Design review of the part built by this model. Coordinates are the model's own, in mm. Round coordinates to 2 decimals unless told otherwise and drop trailing zeros. Loops run counter-clockwise (first coordinate to the right, second up) from the corner with the lowest first, then second, coordinate; pieces in that order, holes last. Notation, with made-up numbers: (35, 45.25) -> (49, 45.25) arc R21 cw to (49, 58.25) -> close; hole circle Ø4 at (19, 44). An arc over 180 degrees is marked (long way). Use a Markdown table: item, result. Add a question column.
from build123d import *

# Parameters (mm, degrees)
BOSS_EXTRUDE1_DEPTH = 3
SKETCH2_R           = 1.5
SKETCH2_R_2         = 1.35
CUT_EXTRUDE1_DEPTH  = 25
CHAMFER1_SIZE       = 14


with BuildPart() as part:
    # Sketch1 → Boss-Extrude1 (new body)
    with BuildSketch(Plane(origin=(0, 0, 0), x_dir=(1, 0, 0), z_dir=(0, 1, 0))):
        Polygon((19.120621977, 112.5), (28.120621977, 112.5), (28.120621977, -112.5), (-49.879378023, -112.5), (-49.879378023, 112.5), (-40.879378023, 112.5), (-40.879378023, 122.5), (19.120621977, 122.5), align=None)
    extrude(amount=BOSS_EXTRUDE1_DEPTH)

    # Sketch2 → Cut-Extrude1 (cut)
    with BuildSketch(Plane(origin=(0, 3, 0), x_dir=(1, 0, 0), z_dir=(0, 1, 0))):
        with Locations(Location((14.120621977, 107.5, 0), (0, 0, 270))):
            Circle(SKETCH2_R)
        with Locations(Location((-35.879378023, 107.5, 0), (0, 0, 270))):
            Circle(SKETCH2_R)
        with Locations(Location((-30.879378023, -107.5, 0), (0, 0, 270))):
            Circle(SKETCH2_R)
        with Locations(Location((9.120621977, -107.5, 0), (0, 0, 270))):
            Circle(SKETCH2_R)
        with Locations(Location((-35.379378023, -82.5, 0), (0, 0, 270))):
            Circle(SKETCH2_R_2)
        with Locations(Location((13.620621977, -82.5, 0), (0, 0, 270))):
            Circle(SKETCH2_R_2)
        with Locations(Location((-35.379378023, -24.5, 0), (0, 0, 270))):
            Circle(SKETCH2_R_2)
        with Locations(Location((13.620621977, -24.5, 0), (0, 0, 270))):
            Circle(SKETCH2_R_2)
        with Locations(Location((-19.879378023, -105, 0), (0, 0, 270))):
            Circle(SKETCH2_R_2)
        with Locations(Location((-1.879378023, -105, 0), (0, 0, 270))):
            Circle(SKETCH2_R_2)
        with Locations(Location((-19.879378023, -95, 0), (0, 0, 270))):
            Circle(SKETCH2_R_2)
        with Locations(Location((-1.879378023, -95, 0), (0, 0, 270))):
            Circle(SKETCH2_R_2)
    extrude(amount=-CUT_EXTRUDE1_DEPTH, mode=Mode.SUBTRACT)

    # Chamfer1
    chamfer1_edges = [part.edges().sort_by_distance(p)[0] for p in [
        (28.120621977, 1.5, 112.5),
        (-49.879378023, 1.5, 112.5),
    ]]
    chamfer(chamfer1_edges, length=CHAMFER1_SIZE)


solid = part.part
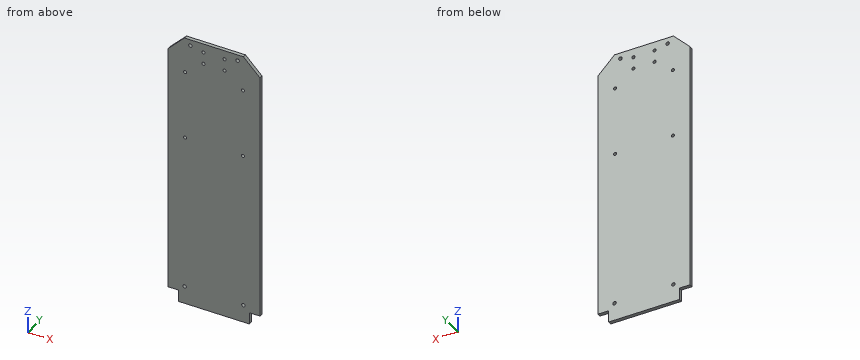
1. Consider section B-B on x = 23.5. State the section outline as (y, z) points.
2. Consider section A-A on y = 1.25. Give the number of separate pieces and of enclosed holes in the cut face, plus the area to 3 significant figures.
3. Insertion check: P1, Ø0.9, axis at y = 1.5, z = -118.5, coming from the +X side. The pin has a flat end and moves straight along its axis. Give the tip position at first contact, or say it passes through.
4. To check wall thickness, follow probe 1 along X at (y, z) = (0.75, 107.5); probe 2 along Z at (x, y) = (-20, 1); probe 3 along X at (y, z) = (1.1, 24.5). State the ranges of each line that lie inside material, in increasing order. Write a range as from..to.
Verdict:
| question | item | result |
|---|---|---|
| 1 | outline | (0, -112.5) -> (3, -112.5) -> (3, 103.12) -> (0, 103.12) -> close |
| 2 | separate pieces | 1 |
| 2 | enclosed holes | 12 |
| 2 | area | 17,900 mm² |
| 3 | P1 | stops at x = 19.12 |
| 4 | probe 1 | x = -40.88..-32.38, -29.38..7.62, 10.62..19.12 |
| 4 | probe 2 | z = -122.5..93.66, 96.34..103.66, 106.34..112.5 |
| 4 | probe 3 | x = -49.88..-36.73, -34.03..12.27, 14.97..28.12 |
